```python
from build123d import *

# Parameters (mm, degrees)
SKETCH1_W           = 281
SKETCH1_H           = 229
SKETCH1_R           = 2.5
SKETCH1_R_2         = 2
SKETCH1_R_3         = 1.95
SKETCH1_W_2         = 12.5
SKETCH1_H_2         = 4.6
SKETCH1_W_3         = 15
SKETCH1_W_4         = 4.6
SKETCH1_H_3         = 20
SKETCH1_W_5         = 20
BOSS_EXTRUDE1_DEPTH = 4.6
SKETCH2_W           = 281
SKETCH2_H           = 229
SKETCH2_W_2         = 279
SKETCH2_H_2         = 227
CUT_EXTRUDE1_DEPTH  = 182.305432903
SKETCH3_W           = 25
SKETCH3_H           = 5
CUT_EXTRUDE2_DEPTH  = 180.899027235
SKETCH6_W           = 2.5
SKETCH6_H           = 12
CUT_EXTRUDE5_DEPTH  = 180.899027235
CUT_EXTRUDE4_DEPTH  = 180.899027235
SKETCH8_W           = 2
SKETCH8_H           = 27.99999988
CUT_EXTRUDE7_DEPTH  = 180.899027235
FILLET2_R           = 0.5


with BuildPart() as part:
    # Sketch1 → Boss-Extrude1 (new body)
    with BuildSketch(Plane(origin=(0, 0, 0), x_dir=(1, 0, 0), z_dir=(0, 1, 0))):
        Rectangle(SKETCH1_W, SKETCH1_H)
        with Locations(Location((-134.5, 108.5, 0), (0, 0, 270))):
            Circle(SKETCH1_R, mode=Mode.SUBTRACT)
        with Locations(Location((134.5, 108.5, 0), (0, 0, 270))):
            Circle(SKETCH1_R, mode=Mode.SUBTRACT)
        with Locations(Location((83.5, 108.5, 0), (0, 0, 270))):
            Circle(SKETCH1_R, mode=Mode.SUBTRACT)
        with Locations(Location((134.5, -108.5, 0), (0, 0, 270))):
            Circle(SKETCH1_R, mode=Mode.SUBTRACT)
        with Locations(Location((83.5, -56.5, 0), (0, 0, 270))):
            Circle(SKETCH1_R, mode=Mode.SUBTRACT)
        with Locations(Location((-134.5, -56.5, 0), (0, 0, 270))):
            Circle(SKETCH1_R, mode=Mode.SUBTRACT)
        with Locations(Location((101.3, 7.23, 0), (0, 0, 270))):
            Circle(SKETCH1_R_2, mode=Mode.SUBTRACT)
        with Locations(Location((-134.5, -108.5, 0), (0, 0, 270))):
            Circle(SKETCH1_R, mode=Mode.SUBTRACT)
        with Locations(Location((131.3, 7.23, 0), (0, 0, 270))):
            Circle(SKETCH1_R_2, mode=Mode.SUBTRACT)
        with Locations(Location((-21.75, -104.5, 0), (0, 0, 270))):
            Circle(SKETCH1_R_3, mode=Mode.SUBTRACT)
        with Locations(Location((-29.25, -93.5, 0), (0, 0, 270))):
            Circle(SKETCH1_R_3, mode=Mode.SUBTRACT)
        with Locations(Location((-21.75, -76.5, 0), (0, 0, 270))):
            Circle(SKETCH1_R_3, mode=Mode.SUBTRACT)
        with Locations((-122.75, -63.8)):
            Rectangle(SKETCH1_W_2, SKETCH1_H_2, mode=Mode.SUBTRACT)
        with Locations((116.3, 43.7)):
            Rectangle(SKETCH1_W_3, SKETCH1_H_2, mode=Mode.SUBTRACT)
        with Locations((116.3, -13.2)):
            Rectangle(SKETCH1_W_3, SKETCH1_H_2, mode=Mode.SUBTRACT)
        with Locations((90.8, -31.5)):
            Rectangle(SKETCH1_W_4, SKETCH1_H_3, mode=Mode.SUBTRACT)
        with Locations((90.8, 78.5)):
            Rectangle(SKETCH1_W_4, SKETCH1_H_3, mode=Mode.SUBTRACT)
        with Locations((-66.5, -63.8)):
            Rectangle(SKETCH1_W_5, SKETCH1_H_2, mode=Mode.SUBTRACT)
        with Locations((53.5, -63.8)):
            Rectangle(SKETCH1_W_5, SKETCH1_H_2, mode=Mode.SUBTRACT)
        with Locations((90.8, 23.5)):
            Rectangle(SKETCH1_W_4, SKETCH1_H_3, mode=Mode.SUBTRACT)
        with Locations((-6.5, -63.8)):
            Rectangle(SKETCH1_W_5, SKETCH1_H_2, mode=Mode.SUBTRACT)
    extrude(amount=BOSS_EXTRUDE1_DEPTH)

    # Sketch2 → Cut-Extrude1 (cut, through all)
    with BuildSketch(Plane(origin=(0, 4.6, 0), x_dir=(1, 0, 0), z_dir=(0, 1, 0))):
        Rectangle(SKETCH2_W, SKETCH2_H)
        Rectangle(SKETCH2_W_2, SKETCH2_H_2, mode=Mode.SUBTRACT)
    extrude(amount=-CUT_EXTRUDE1_DEPTH, mode=Mode.SUBTRACT)

    # Sketch3 → Cut-Extrude2 (cut, through all)
    with BuildSketch(Plane.XZ):
        with Locations((106.5, 64)):
            Rectangle(SKETCH3_W, SKETCH3_H)
    extrude(amount=-CUT_EXTRUDE2_DEPTH, mode=Mode.SUBTRACT)

    # Sketch6 → Cut-Extrude5 (cut, through all)
    with BuildSketch(Plane(origin=(0, 4.6, 0), x_dir=(1, 0, 0), z_dir=(0, 1, 0))):
        with Locations((64.25, -78)):
            Rectangle(SKETCH6_W, SKETCH6_H)
        with Locations((64.25, -97.5)):
            Rectangle(SKETCH6_W, SKETCH6_H)
    extrude(amount=-CUT_EXTRUDE5_DEPTH, mode=Mode.SUBTRACT)

    # Sketch5 → Cut-Extrude4 (cut, through all)
    with BuildSketch(Plane(origin=(0, 0, 0), x_dir=(1, 0, 0), z_dir=(0, 1, 0))):
        with BuildLine():
            Line((132, -75.5), (132, -94.5))
            ThreePointArc((132, -94.5), (129.5, -97), (127, -94.5))
            Line((127, -94.5), (127, -75.5))
            ThreePointArc((127, -75.5), (129.5, -73), (132, -75.5))
        make_face()
        with BuildLine():
            Line((122, -75.5), (122, -94.5))
            ThreePointArc((122, -94.5), (119.5, -97), (117, -94.5))
            Line((117, -94.5), (117, -75.5))
            ThreePointArc((117, -75.5), (119.5, -73), (122, -75.5))
        make_face()
        with BuildLine():
            Line((112, -75.5), (112, -94.5))
            ThreePointArc((112, -94.5), (109.5, -97), (107, -94.5))
            Line((107, -94.5), (107, -75.5))
            ThreePointArc((107, -75.5), (109.5, -73), (112, -75.5))
        make_face()
        with BuildLine():
            Line((102, -75.5), (102, -94.5))
            ThreePointArc((102, -94.5), (99.5, -97), (97, -94.5))
            Line((97, -94.5), (97, -75.5))
            ThreePointArc((97, -75.5), (99.5, -73), (102, -75.5))
        make_face()
        with BuildLine():
            Line((92, -75.5), (92, -94.5))
            ThreePointArc((92, -94.5), (89.5, -97), (87, -94.5))
            Line((87, -94.5), (87, -75.5))
            ThreePointArc((87, -75.5), (89.5, -73), (92, -75.5))
        make_face()
    extrude(amount=CUT_EXTRUDE4_DEPTH, mode=Mode.SUBTRACT)

    # Sketch8 → Cut-Extrude7 (cut, through all)
    with BuildSketch(Plane(origin=(0, 4.6, 0), x_dir=(1, 0, 0), z_dir=(0, 1, 0))):
        with Locations((128.26444081, -47.0000889)):
            Rectangle(SKETCH8_W, SKETCH8_H)
    extrude(amount=-CUT_EXTRUDE7_DEPTH, mode=Mode.SUBTRACT)

    # Fillet2
    fillet2_edges = [part.edges().sort_by_distance(p)[0] for p in [
        (-139.5, 2.3, -113.5),
        (139.5, 2.3, -113.5),
        (139.5, 2.3, 113.5),
        (-139.5, 2.3, 113.5),
    ]]
    fillet(fillet2_edges, radius=FILLET2_R)


solid = part.part
```
The model under review builds one solid part; all positions refer to its coordinate system, in mm. Give positions to 0.01 mm unless a question says otherwise; leave off trailing zeros. Loops run counter-clockwise (first coordinate to the right, second up) from the corner with the lowest first, then second, coordinate; pieces in that order, holes last. Notation, with made-up numbers: (37.25, 68) - (83.25, 68) arc R6 cw to (83.25, 78) - close; hole circle Ø8 at (34.25, 64). An arc over 180 degrees is marked (long way). Answer as a JSON object with one key per item and string values.
Q1. To check wall thickness, follow line 1 along Z through (x, y) = (-134.5, 1.6); line 2 along Z through (x, y) = (134.5, 2.05); line 3 along X through (y, z) = (2.4, 26). State the ranges of each line that lie inside material, in increasing order.
Worked out:
{"line 1": "z = -113.5 to -111, -106 to 54, 59 to 106, 111 to 113.5", "line 2": "z = -113.5 to -111, -106 to 106, 111 to 113.5", "line 3": "x = -139.5 to 88.5, 93.1 to 139.5"}
Q2. Add section B-B on y = 3.9. Count the separate pieces of the cut face and the enclosed holes in it, plus the area to 3 significant figures.
Worked out:
{"separate pieces": "1", "enclosed holes": "30", "area": "61,600 mm^2"}
Q3. Add section A-A on z = -21. State the section outline as (x, y) points, plus the area to 3 significant figures.
Worked out:
{"outline": "(-139.5, 0) - (88.5, 0) - (88.5, 4.6) - (-139.5, 4.6) - close; (93.1, 0) - (139.5, 0) - (139.5, 4.6) - (93.1, 4.6) - close", "area": "1,260 mm^2"}
